Check sheet for the drawn part. Datum: minimum x, y, z corner. Units: mm. Coordinates: 2 decimals unless noted, no trailing zeros. Order: outer loops, then holes, each group sorted by start corner. A loop starts at its lowest first (then second) coordinate and runs counter-clockwise, first axis right, second up.
1. Cross-section at B-B (x = 41). Enter the section's corners in (y, z).
2. Thickness scan on line 1 (X direction, y = 12.75, z = 2); line 2 (Y direction, x = 13, z = 2); line 3 (Y direction, x = 41.5, z = 1.5). Record the ranges inside material, lowest first.
3. Cross-section at A-A (y = 14.25). Enter the section's corners in (x, z), then the cut area to 3 significant figures.
4. Cross-section at D-D (y = 4). Enter the section's corners in (x, z), then the cut area to 3 significant figures.
5. Cross-section at C-C (z = 1.5). Count the separate pieces of the cut face and the enclosed holes in it, then the cut area to 3 significant figures.
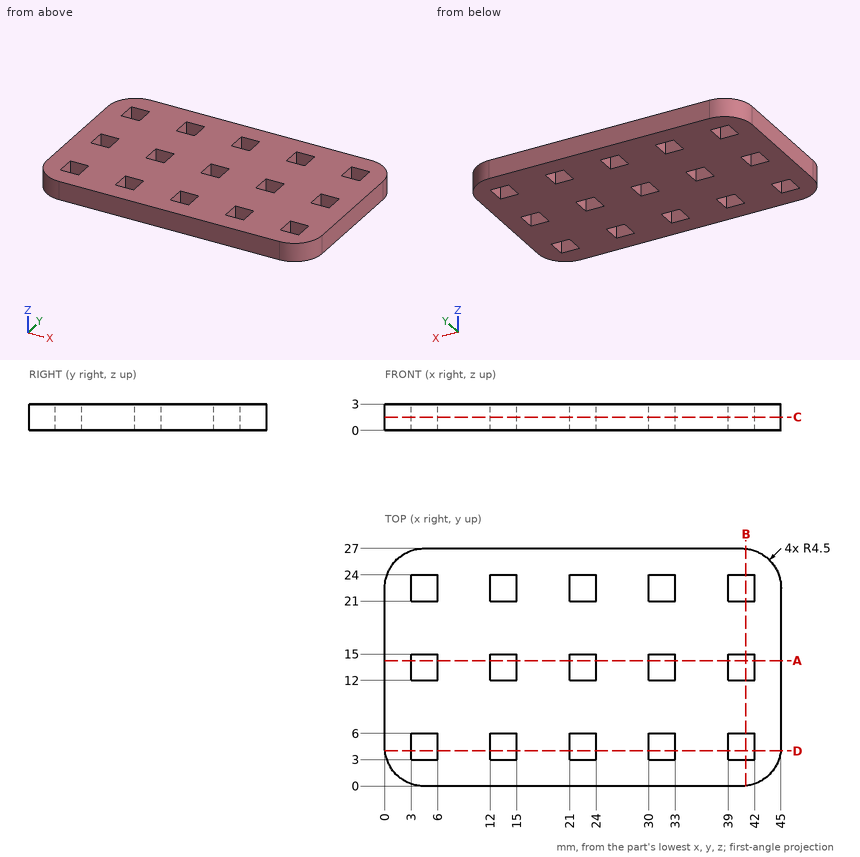
Data:
1. outline: (0.03, 0) - (3, 0) - (3, 3) - (0.03, 3) - close; (6, 0) - (12, 0) - (12, 3) - (6, 3) - close; (15, 0) - (21, 0) - (21, 3) - (15, 3) - close; (24, 0) - (26.97, 0) - (26.97, 3) - (24, 3) - close
2. line 1: x = 0 to 3, 6 to 12, 15 to 21, 24 to 30, 33 to 39, 42 to 45
2. line 2: y = 0 to 3, 6 to 12, 15 to 21, 24 to 27
2. line 3: y = 0.11 to 3, 6 to 12, 15 to 21, 24 to 26.89
3. outline: (0, 0) - (3, 0) - (3, 3) - (0, 3) - close; (6, 0) - (12, 0) - (12, 3) - (6, 3) - close; (15, 0) - (21, 0) - (21, 3) - (15, 3) - close; (24, 0) - (30, 0) - (30, 3) - (24, 3) - close; (33, 0) - (39, 0) - (39, 3) - (33, 3) - close; (42, 0) - (45, 0) - (45, 3) - (42, 3) - close
3. area: 90.0 mm2
4. outline: (0.03, 0) - (3, 0) - (3, 3) - (0.03, 3) - close; (6, 0) - (12, 0) - (12, 3) - (6, 3) - close; (15, 0) - (21, 0) - (21, 3) - (15, 3) - close; (24, 0) - (30, 0) - (30, 3) - (24, 3) - close; (33, 0) - (39, 0) - (39, 3) - (33, 3) - close; (42, 0) - (44.97, 0) - (44.97, 3) - (42, 3) - close
4. area: 89.8 mm2
5. separate pieces: 1
5. enclosed holes: 15
5. area: 1,060 mm2
